Can you work these out from the drawing? Everything is in mm from the part's minimum corner. Round coordinates to 2 decimals unless told otherwise and drop trailing zeros. Loops run counter-clockwise (first coordinate to the right, second up) from the corner with the lowest first, then second, coordinate; pieces in that order, holes last. Notation, with made-up numbers: (-12, 31) -> (21, 31) arc R18 cw to (21, 66) -> close; hole circle Ø1 at (84.25, -20). An arc over 180 degrees is marked (long way). One line per item, written item: value.
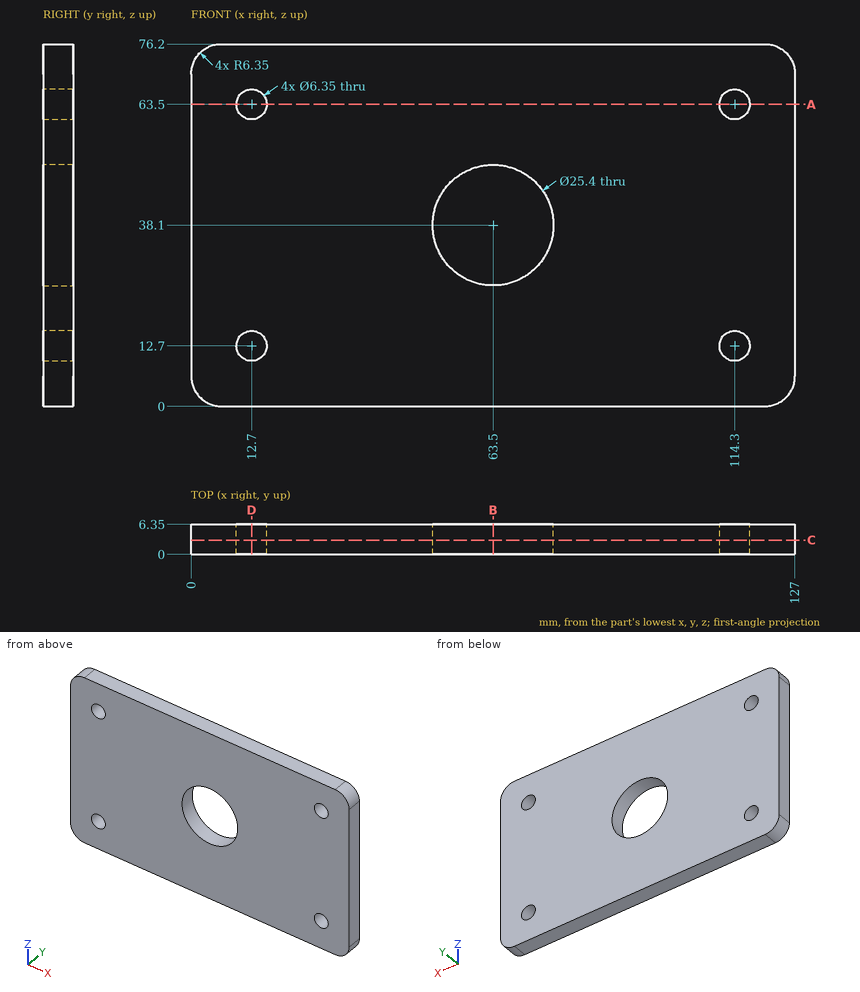
(1) Please list where these lines run through material, in increasing order: L1, parallel to X at y = 5, z = 63.5 (3 decimals); L2, parallel to X at y = 0.5, z = 11; L3, parallel to Z at x = 111.5, y = 1.75.
Results below:
L1: x = 0 to 9.525, 15.875 to 111.125, 117.475 to 127
L2: x = 0 to 10.02, 15.38 to 111.62, 116.98 to 127
L3: z = 0 to 11.2, 14.2 to 62, 65 to 76.2
(2) Imagine slicing it at B-B on x = 63.5. Write out the boundary of the cut face in (y, z), then the cut area to 3 significant figures.
Results below:
outline: (0, 0) -> (6.35, 0) -> (6.35, 25.4) -> (0, 25.4) -> close; (0, 50.8) -> (6.35, 50.8) -> (6.35, 76.2) -> (0, 76.2) -> close
area: 323 mm²
(3) Imagine slicing it at A-A on z = 63.5. Write out the boundary of the cut face in (x, y) (3 decimals), then the cut area to 3 significant figures.
Results below:
outline: (0, 0) -> (9.525, 0) -> (9.525, 6.35) -> (0, 6.35) -> close; (15.875, 0) -> (111.125, 0) -> (111.125, 6.35) -> (15.875, 6.35) -> close; (117.475, 0) -> (127, 0) -> (127, 6.35) -> (117.475, 6.35) -> close
area: 726 mm²
(4) Imagine slicing it at C-C on y = 3. Write out the boundary of the cut face in (x, z) (3 decimals).
Results below:
outline: (0, 6.35) arc R6.35 ccw to (6.35, 0) -> (120.65, 0) arc R6.35 ccw to (127, 6.35) -> (127, 69.85) arc R6.35 ccw to (120.65, 76.2) -> (6.35, 76.2) arc R6.35 ccw to (0, 69.85) -> close; hole circle Ø6.35 at (12.7, 12.7); hole circle Ø6.35 at (12.7, 63.5); hole circle Ø25.4 at (63.5, 38.1); hole circle Ø6.35 at (114.3, 12.7); hole circle Ø6.35 at (114.3, 63.5)
(5) Imagine slicing it at D-D on x = 12.7. Write out the boundary of the cut face in (y, z) (3 decimals).
Results below:
outline: (0, 0) -> (6.35, 0) -> (6.35, 9.525) -> (0, 9.525) -> close; (0, 15.875) -> (6.35, 15.875) -> (6.35, 60.325) -> (0, 60.325) -> close; (0, 66.675) -> (6.35, 66.675) -> (6.35, 76.2) -> (0, 76.2) -> close
